The model under review builds one solid part; all positions refer to its coordinate system, in mm. A direction names the side the tool comes from. Coordinates: 2 decimals unless noted, no trailing zeros. Loops run counter-clockwise (first coordinate to the right, second up) from the corner with the lowest first, then second, coordinate; pieces in that order, holes last. Notation, with made-up numbers: M 27,-19 L 41,-19 A5 ccw 41,-15 Z; hole C 8.5,52.25 d3. An arc over 180 degrees is marked long. Return JSON: item names as keys, results as strings.
```python
from build123d import *

# Parameters (mm, degrees)
F1_DEPTH = 1.27
F2_R     = 6.35
F3_DEPTH = 25.4
F4_W     = 12.6276115155
F4_H     = 1.524
F5_DEPTH = 25.4
F6_R     = 1.8415
F8_DEPTH = 25.4
F9_R     = 2.53999


# Not quite as in the source:
# - a fillet or chamfer is up to 0.001 mm smaller than in the source, because OpenCascade refuses the exact size


with BuildPart() as f1:
    # F0 (on Top) → F1 (new body, symmetric)
    with BuildSketch(Plane.XY):
        with BuildLine():
            ThreePointArc((-11.118852542, -6.35), (-9.4633932444, -3.3649028089), (-8.89, 0))
            ThreePointArc((-8.89, 0), (-9.4633932444, 3.3649028089), (-11.118852542, 6.35))
            ThreePointArc((-11.118852542, 6.35), (-29.21, 0), (-11.118852542, -6.35))
        make_face()
        with BuildLine():
            ThreePointArc((-11.118852542, 6.35), (-9.4633932444, 3.3649028089), (-8.89, 0))
            ThreePointArc((-8.89, 0), (-9.4633932444, -3.3649028089), (-11.118852542, -6.35))
            Line((-11.118852542, -6.35), (11.118852542, -6.35))
            ThreePointArc((11.118852542, -6.35), (8.89, 0), (11.118852542, 6.35))
            Line((11.118852542, 6.35), (-11.118852542, 6.35))
        make_face()
        with BuildLine():
            ThreePointArc((29.21, 0), (22.4149028089, 9.5866067556), (11.118852542, 6.35))
            ThreePointArc((11.118852542, 6.35), (8.89, 0), (11.118852542, -6.35))
            ThreePointArc((11.118852542, -6.35), (22.4149028089, -9.5866067556), (29.21, 0))
        make_face()
    extrude(amount=F1_DEPTH, both=True)

    # F2 (on face) → F3 (cut)
    with BuildSketch(Plane.XY.offset(1.27)):
        with Locations((-19.05, 0)):
            Circle(F2_R)
        with Locations((19.05, 0)):
            Circle(F2_R)
    extrude(amount=-F3_DEPTH, mode=Mode.SUBTRACT)

    # F4 (on face) → F5 (cut)
    with BuildSketch(Plane.XY.offset(1.27)):
        with Locations((-22.8961942422, 0)):
            Rectangle(F4_W, F4_H)
        with Locations((22.8961942422, 0)):
            Rectangle(F4_W, F4_H)
    extrude(amount=-F5_DEPTH, mode=Mode.SUBTRACT)

    # F6
    f6_edges = [f1.edges().sort_by_distance(p)[0] for p in [
        (-29.181385, 0.762, 0),
        (-25.354114, 0.762, 0),
        (-25.354114, -0.762, 0),
        (-29.181385, -0.762, 0),
        (25.354114, -0.762, 0),
        (25.354114, 0.762, 0),
        (29.181385, 0.762, 0),
        (29.181385, -0.762, 0),
        (-11.118853, -6.35, 0),
        (11.118853, -6.35, 0),
        (11.118853, 6.35, 0),
        (-11.118853, 6.35, 0),
    ]]
    fillet(f6_edges, radius=F6_R)

    # F7 (on face) → F8 (cut)
    with BuildSketch(Plane.XY.offset(1.27)):
        with BuildLine():
            ThreePointArc((-9.2126223006, 2.54), (-8.89, 0), (-9.2126223006, -2.54))
            Line((-9.2126223006, -2.54), (9.2126223006, -2.54))
            ThreePointArc((9.2126223006, -2.54), (8.89, 0), (9.2126223006, 2.54))
            Line((9.2126223006, 2.54), (-9.2126223006, 2.54))
        make_face()
    extrude(amount=-F8_DEPTH, mode=Mode.SUBTRACT)

    # F9 (radius 2.54 in the source; OpenCascade refuses exactly that, so slightly less here)
    f9_edges = [f1.edges().sort_by_distance(p)[0] for p in [
        (-9.212622, -2.54, 0),
        (-9.212622, 2.54, 0),
        (9.212622, 2.54, 0),
        (9.212622, -2.54, 0),
    ]]
    fillet(f9_edges, radius=F9_R)


solid = f1.part
```
1. Machinability: for faces 1 (the face through (-28.428, -1.505, 0.018)), 2 (the face through (0, -4, -1.27)), 3 (the face through (-8.166, -1.776, -0.018)), 4 (the face through (11.022, 6.507, -0.018)), 5 (the face through (-11.022, -6.507, 0.018)), which of the approach directions +Z, -Z, +X, -X, +Y, -Y give a long, thin tool a straight path to every point of the face, cutting with its end or side? Answer none if there is none.
Check values:
{"face 1": "+Z, -Z, -X", "face 2": "-Z, +X, -X, +Y, -Y", "face 3": "+Z, -Z", "face 4": "+Z, -Z, +Y", "face 5": "+Z, -Z, -Y"}
2. The part is to be moulded in two halves that separate along X. For faces 6 (the face through (28.457, -1.544, -0.018)), 7 (the face through (-28.457, 1.544, 0.018)), 8 (the face through (11.003, -6.498, -0.018)), say which applies: released by +X, released by -X, zero draft, split by the parting line, or undercut.
Check values:
{"face 6": "released by +X", "face 7": "released by -X", "face 8": "undercut"}
3. Add section C-C on y = -7.5. Give the boundary of the cut face in (x, z).
Check values:
{"outline": "M -25.9,-1.27 L -12.2,-1.27 L -12.2,1.27 L -25.9,1.27 Z; M 12.2,-1.27 L 25.9,-1.27 L 25.9,1.27 L 12.2,1.27 Z"}
4. Insertion check: pin 1 Ø1 at (y, z) = (0.5, -0.5) entering from -X; pin 2 Ø0.8 at (x, z) = (-1.5, 0.5) entering from +Y; pin 3 Ø0.8 at (x, z) = (2.5, 0) entering from -Y. Each pin has a flat end and moves straight along its axis. Give the tip position at first contact, or say it passes through.
Check values:
{"pin 1": "x = -27.86", "pin 2": "y = 6.35", "pin 3": "y = -6.35"}
5. To check wall thickness, follow line 1 (Y direction, x = -19.05, z = -0.2); line 2 (X direction, y = -5, z = 0.35); line 3 (X direction, y = -4.75, z = -0.65). State the ranges of each line that lie inside material, in increasing order.
Check values:
{"line 1": "-10.16 to -6.35, 6.35 to 10.16", "line 2": "-27.89 to -22.96, -15.14 to 15.14, 22.96 to 27.89", "line 3": "-28.03 to -23.26, -14.84 to 14.84, 23.26 to 28.03"}
6. Add section A-A on x = -5. Give the boundary of the cut face in (y, z), plus the area to 3 significant figures.
Check values:
{"outline": "M -6.35,-1.27 L -2.54,-1.27 L -2.54,1.27 L -6.35,1.27 Z; M 2.54,-1.27 L 6.35,-1.27 L 6.35,1.27 L 2.54,1.27 Z", "area": "19.4 mm²"}
